Could you check a few things on this model? Use its own coordinates, in mm. Coordinates: 2 decimals unless noted, no trailing zeros. Loops run counter-clockwise (first coordinate to the right, second up) from the corner with the lowest first, then second, coordinate; pieces in that order, holes last.
1) Imagine slicing it at A-A on z = 1.75. Please give me the cut outline in (x, y).
2) Imagine slicing it at D-D on z = -2.5. Please give me the cut outline in (x, y), plus the area to 3 significant figures.
3) Imagine slicing it at B-B on x = 0. Please give me the cut outline in (y, z) (3 decimals), plus the area to 3 significant figures.
4) Thinking about a two-plate mould opening in Z: for faces 1 (the face through (1.89, -1.25, -0.25)), 2 (the face through (0, -1, -3.556)), 3 (the face through (-3.094, -1.252, 1.753)), which applies, released by +Z, released by -Z, zero draft, split by the parting line, or undercut?
5) If I drill on line 1 along Z through (x, y) = (0.5, -2); line 2 along X through (y, z) = (-2.1, 0.5); line 3 along Z through (x, y) = (-1.5, -1.45), over which ranges is the centre line in solid material (lowest first)?
6) Imagine slicing it at C-C on y = -1. Please give me the cut outline in (x, z) (3 decimals).
7) Will these pins go through, and if not, where does the flat tip stop? P1, Ø3, axis at x = 0, z = 0, coming from the +Y side; P2, Ø2, axis at x = -1.5, z = -1, coming from the -Y side.
```python
from build123d import *

# Parameters (mm, degrees)
SKETCH1_R           = 1.905
BOSS_EXTRUDE1_DEPTH = 2.54


with BuildPart() as part:
    # Sketch1 → Boss-Extrude1 (new body)
    with BuildSketch(Plane(origin=(0, 0, 0), x_dir=(1, 0, 0), z_dir=(0, 1, 0))):
        Polygon((2.053057557, 3.556), (-2.053057557, 3.556), (-4.106115114, 0), (-2.053057557, -3.556), (2.053057557, -3.556), (4.106115114, 0), align=None)
        with Locations(Location((0, 0, 0), (0, 0, 270))):
            Circle(SKETCH1_R, mode=Mode.SUBTRACT)
    extrude(amount=-BOSS_EXTRUDE1_DEPTH)


solid = part.part
```
Filled in:
1. outline: (-3.1, -2.54) - (-0.75, -2.54) - (-0.75, 0) - (-3.1, 0) - close; (0.75, -2.54) - (3.1, -2.54) - (3.1, 0) - (0.75, 0) - close
2. outline: (-2.66, -2.54) - (2.66, -2.54) - (2.66, 0) - (-2.66, 0) - close
2. area: 13.5 mm2
3. outline: (-2.54, -3.556) - (0, -3.556) - (0, -1.905) - (-2.54, -1.905) - close; (-2.54, 1.905) - (0, 1.905) - (0, 3.556) - (-2.54, 3.556) - close
3. area: 8.39 mm2
4. face 1: undercut
4. face 2: released by -Z
4. face 3: released by +Z
5. line 1: z = -3.56 to -1.84, 1.84 to 3.56
5. line 2: x = -3.82 to -1.84, 1.84 to 3.82
5. line 3: z = -3.56 to -1.17, 1.17 to 3.56
6. outline: (-4.106, 0) - (-2.053, -3.556) - (2.053, -3.556) - (4.106, 0) - (2.053, 3.556) - (-2.053, 3.556) - close; hole circle Ø3.81 at (0, 0)
7. P1: passes through
7. P2: stops at y = -2.54
